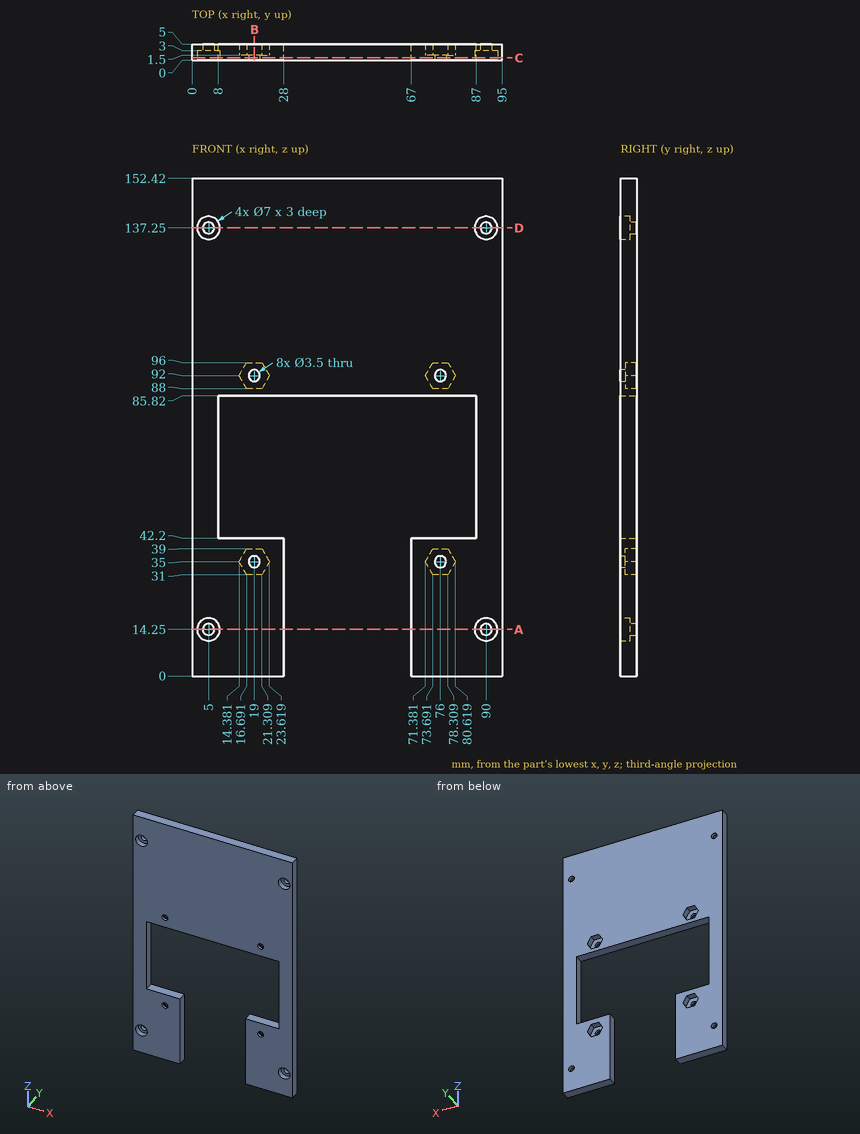
Geometry check sheet. Reference: drawing and pictorial views, mm from the part's lowest x, y, z. Round coordinates to 2 decimals unless told otherwise and drop trailing zeros. Write each loop counter-clockwise with the first axis right and the second up, starting at its lowest first coordinate (ties: lowest second). Pieces come first, ordered by that corner, then holes.
Item 1: Section check A-A (z = 14.25). Record the boundary of the cut face in (x, y), plus the area to 3 significant figures.
Determined:
outline: (0, 0) - (1.5, 0) - (1.5, 3) - (3.25, 3) - (3.25, 5) - (0, 5) - close; (6.75, 3) - (8.5, 3) - (8.5, 0) - (28, 0) - (28, 5) - (6.75, 5) - close; (67, 0) - (86.5, 0) - (86.5, 3) - (88.25, 3) - (88.25, 5) - (67, 5) - close; (91.75, 3) - (93.5, 3) - (93.5, 0) - (95, 0) - (95, 5) - (91.75, 5) - close
area: 224 mm2
Item 2: Section check B-B (x = 19). Record the boundary of the cut face in (y, z).
Determined:
outline: (0, 0) - (5, 0) - (5, 31) - (1.5, 31) - (1.5, 33.25) - (0, 33.25) - close; (0, 36.75) - (1.5, 36.75) - (1.5, 39) - (5, 39) - (5, 42.2) - (0, 42.2) - close; (0, 85.82) - (5, 85.82) - (5, 88) - (1.5, 88) - (1.5, 90.25) - (0, 90.25) - close; (0, 93.75) - (1.5, 93.75) - (1.5, 96) - (5, 96) - (5, 152.42) - (0, 152.42) - close
Item 3: Section check D-D (z = 137.25). Record the boundary of the cut face in (x, y).
Determined:
outline: (0, 0) - (1.5, 0) - (1.5, 3) - (3.25, 3) - (3.25, 5) - (0, 5) - close; (6.75, 3) - (8.5, 3) - (8.5, 0) - (86.5, 0) - (86.5, 3) - (88.25, 3) - (88.25, 5) - (6.75, 5) - close; (91.75, 3) - (93.5, 3) - (93.5, 0) - (95, 0) - (95, 5) - (91.75, 5) - close
Item 4: Material ranges on line 1 along X through (y, z) = (1.1, 137.25); line 2 along Z through (x, y) = (76, 0.6); line 3 along Z through (x, y) = (84, 4.15), recorded low to high.
Determined:
line 1: x = 0 to 1.5, 8.5 to 86.5, 93.5 to 95
line 2: z = 0 to 33.25, 36.75 to 42.2, 85.82 to 90.25, 93.75 to 152.42
line 3: z = 0 to 42.2, 85.82 to 152.42
Item 5: Section check C-C (y = 0.75). Give the number of separate pieces and of enclosed holes in the cut face.
Determined:
separate pieces: 1
enclosed holes: 8
Item 6: Go/stop test with flat-tipped pins: pin 1 Ø5.5 at (x, z) = (88.5, 14) entering from -Y; pin 2 Ø2.5 at (x, y) = (42.5, 2) entering from -Z; pin 3 Ø4.5 at (x, z) = (5, 14.25) entering from -Y; pin 4 Ø4 at (x, z) = (75.5, 34) entering from +Y. Record where each tip stops, or that it passes through.
Determined:
pin 1: stops at y = 0
pin 2: stops at z = 85.82
pin 3: stops at y = 3
pin 4: stops at y = 1.5
